Could you check a few things on this model? Use its own coordinates, in mm. Coordinates: 2 decimals unless noted, no trailing zeros. Loops run counter-clockwise (first coordinate to the right, second up) from the corner with the lowest first, then second, coordinate; pieces in that order, holes last. Notation, with made-up numbers: M -3,-0.75 L 56,-0.75 A15 ccw 56,13.25 Z; hole C 51,45 d5. An arc over 180 degrees is marked long. Return JSON: item names as keys, results as strings. Group by question number.
from build123d import *

# Parameters (mm, degrees)
F0_W     = 38.1
F0_H     = 101.6
F0_R     = 6.35
F1_DEPTH = 12.7
F2_R     = 5.08


with BuildPart() as f1:
    # F0 (on Front) → F1 (new body, symmetric)
    with BuildSketch(Plane.XZ):
        Rectangle(F0_W, F0_H)
        with Locations((0, -38.1)):
            Circle(F0_R, mode=Mode.SUBTRACT)
    extrude(amount=F1_DEPTH, both=True)

    # F2
    f2_edges = [f1.edges().sort_by_distance(p)[0] for p in [
        (-19.05, 0, 50.8),
        (19.05, 0, 50.8),
        (19.05, 0, -50.8),
        (-19.05, 0, -50.8),
    ]]
    fillet(f2_edges, radius=F2_R)


solid = f1.part
(1) Imagine slicing it at C-C, the plane y = -4. Write out the boundary of the cut face in (x, z).
(2) Will this pin go through, and if not, where does the flat tip stop? P1, Ø16.5, axis at x = 0, z = -38.1, coming from the -Y side.
(3) Imagine slicing it at B-B, the plane x = 0. Write out the boundary of the cut face in (y, z), then the cut area to 3 significant figures.
(4) We'd pull the mould along X, two halves only. Please class faces 1 (the face through (6.057, 0.178, -36.193)), 2 (the face through (0, 12.7, 1)), 3 (the face through (-17.601, -0.178, -49.272)), 4 (the face through (17.601, -0.178, -49.272)): +X half, -X half, draft (parallel to the pull), parting line (faces both ways), or undercut.
(5) Imagine slicing it at A-A, the plane z = -38.1. Write out the boundary of the cut face in (x, y).
(6) If I drill on L1, parallel to Z at x = 0, y = -7; L2, parallel to Z at x = -1.5, y = 11; L3, parallel to X at y = 10.5, z = -34, over which ranges is the centre line in solid material (lowest first)? Write a range as [from, to].
Checks:
{
 "1": {"outline": "M -19.05,-45.72 A5.08 ccw -13.97,-50.8 L 13.97,-50.8 A5.08 ccw 19.05,-45.72 L 19.05,45.72 A5.08 ccw 13.97,50.8 L -13.97,50.8 A5.08 ccw -19.05,45.72 Z; hole C 0,-38.1 d12.7"},
 "2": {"P1": "y = -12.7"},
 "3": {"outline": "M -12.7,-50.8 L 12.7,-50.8 L 12.7,-44.45 L -12.7,-44.45 Z; M -12.7,-31.75 L 12.7,-31.75 L 12.7,50.8 L -12.7,50.8 Z", "area": "2,260 mm²"},
 "4": {"face 1": "undercut", "face 2": "draft", "face 3": "-X half", "face 4": "+X half"},
 "5": {"outline": "M -19.05,-12.7 L -6.35,-12.7 L -6.35,12.7 L -19.05,12.7 Z; M 6.35,-12.7 L 19.05,-12.7 L 19.05,12.7 L 6.35,12.7 Z"},
 "6": {"L1": "[-50.8, -44.45], [-31.75, 50.8]", "L2": "[-50.8, -44.27], [-31.93, 50.8]", "L3": "[-19.05, -4.85], [4.85, 19.05]"}
}
